Autodesk Inventor part; units mm, degrees
ref_plane "YZ Plane" through (0, 0, 0) normal (1, 0, 0) x (0, 1, 0)
ref_plane "XZ Plane" through (0, 0, 0) normal (0, 1, 0) x (-1, 0, 0)
ref_plane "XY Plane" through (0, 0, 0) normal (0, 0, 1) x (1, 0, 0)
sketch "Sketch1" plane through (0, 0, 0) normal (0, 1, 0) x (-1, 0, 0)
  line L0 (15.6279, 8.093) -> (-18.3721, 8.093)
  line L1 (-18.3721, 8.093) -> (-18.3721, -15.907)
  line L2 (-18.3721, -15.907) -> (15.6279, -15.907)
  line L3 (15.6279, -15.907) -> (15.6279, 8.093)
  point P0 (0, 0)
  dimension "d0" = 24
  dimension "d1" = 34
extrude "Extrusion1" add sketch "Sketch1" along normal blind 4
sketch "Sketch2" plane through (0, 4, 0) normal (0, 1, 0) x (1, 0, 0)
  line L0 (-13.61, -6.4787) -> (16.6862, -6.4787)
  line L1 (16.6862, -6.4787) -> (16.6862, 11.1397)
  line L2 (16.6862, 11.1397) -> (-13.61, 11.1397)
  line L3 (-13.61, 11.1397) -> (-13.61, -6.4787)
  point P0 (0, 0)
extrude "Extrusion2" cut sketch "Sketch2" against normal blind 2.5
sketch "Sketch3" plane through (0, 0, 0) normal (0, -1, 0) x (1, 0, 0)
  line L0 (18.3721, -15.907) -> (-15.6279, -15.907)
  line L1 (18.3721, -15.907) -> (7.3721, -15.907)
  line L2 (7.3721, -15.907) -> (7.3721, -11.907)
  line L3 (7.3721, -11.907) -> (18.3721, -11.907)
  line L4 (18.3721, -11.907) -> (18.3721, -15.907)
  point P0 (0, 0)
  dimension "d6" = 11
  dimension "d7" = 4
extrude "Extrusion3" add sketch "Sketch3" along normal blind 2.5
properties part number "charger"
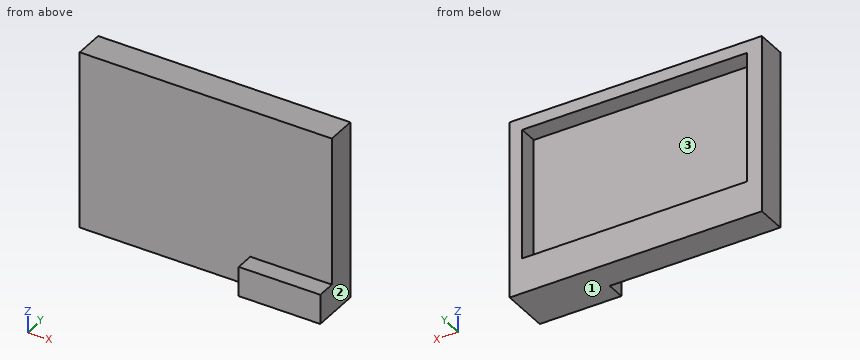
Build history of the part. All positions in model axes, mm. Face numbers are marked on the shaded views. Give positions to 0.01 mm unless a question says otherwise; leave off trailing zeros. Loops run counter-clockwise (first coordinate to the right, second up) from the corner with the lowest first, then second, coordinate; pieces in that order, holes last.
Item 1: Drill centre lines: line 1 (X direction, y = 3.5, z = 5.25); line 2 (Z direction, x = 15, y = 3.5); line 3 (Y direction, x = 11.5, z = 1.25). Where is each one in solid material? Low to high.
Answers follow:
line 1: x = -15.63 to -13.61, 16.69 to 18.37
line 2: z = -15.91 to -11.14, 6.48 to 8.09
line 3: y = 0 to 1.5
Item 2: Slice it at D-D, the plane y = -2. List the corners of the cut face in (x, z).
Answers follow:
outline: (7.37, -15.91) - (18.37, -15.91) - (18.37, -11.91) - (7.37, -11.91) - close
Item 3: Slice it at A-A, the plane y = 2.25. List the corners of the cut face in (x, z).
Answers follow:
outline: (-15.63, -15.91) - (18.37, -15.91) - (18.37, 8.09) - (-15.63, 8.09) - close; hole (-13.61, -11.14) - (16.69, -11.14) - (16.69, 6.48) - (-13.61, 6.48) - close
Item 4: Slice it at B-B, the plane x = 12. List the corners of the cut face in (y, z).
Answers follow:
outline: (-2.5, -15.91) - (4, -15.91) - (4, -11.14) - (1.5, -11.14) - (1.5, 6.48) - (4, 6.48) - (4, 8.09) - (0, 8.09) - (0, -11.91) - (-2.5, -11.91) - close
Item 5: Slice it at C-C, the plane z = -6.5. List the corners of the cut face in (x, y).
Answers follow:
outline: (-15.63, 0) - (18.37, 0) - (18.37, 4) - (16.69, 4) - (16.69, 1.5) - (-13.61, 1.5) - (-13.61, 4) - (-15.63, 4) - close
Item 6: Flat gauge pins, fed straight in: pin 1 (0.8 mm diameter, centred on x = 12, y = -1.5, fed in from +Z); pin 2 (9 mm diameter, centred on x = -4.5, z = 1, fed in from +Y); pin 3 (10 mm diameter, centred on x = 5, z = -3.5, fed in from -Y). Where does each tip first touch, or does it go through?
Answers follow:
pin 1: stops at z = -11.91
pin 2: stops at y = 1.5
pin 3: stops at y = 0
Item 7: Pull direction X, two halves, no side cores. Call the marked faces 1, 2 and 3: released by +X, released by -X, zero draft, split by the parting line, or undercut.
Answers follow:
face 1: zero draft
face 2: released by +X
face 3: undercut
